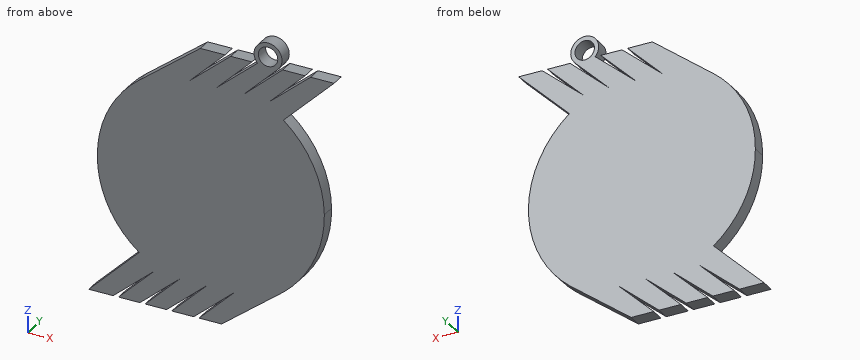
```python
from build123d import *

# Parameters (mm, degrees)
F0_R     = 2.291319
F1_DEPTH = 3.175


with BuildPart() as f1:
    # F0 (on Front) → F1 (new body)
    with BuildSketch(Plane.XZ):
        with BuildLine():
            Line((2.42887, 27.417888), (-3.408971, 27.417888))
            Line((-3.408971, 27.417888), (-17.817384, 16.07928))
            ThreePointArc((-17.817384, 16.07928), (-25.137158, 6.999169), (-27.666417, -4.386364))
            ThreePointArc((-27.666417, -4.386364), (-25.140054, -15.767724), (-17.817384, -24.839458))
            Line((-17.817384, -24.839458), (-29.714837, -36.722033))
            Line((-29.714837, -36.722033), (-23.95565, -36.722033))
            Line((-23.95565, -36.722033), (-14.339792, -28.421288))
            Line((-14.339792, -28.421288), (-22.712222, -36.722033))
            Line((-22.712222, -36.722033), (-17.655194, -36.722033))
            Line((-17.655194, -36.722033), (-8.056328, -28.420344))
            Line((-8.056328, -28.420344), (-16.424194, -36.722033))
            Line((-16.424194, -36.722033), (-11.368304, -36.722033))
            Line((-11.368304, -36.722033), (-1.727521, -28.384091))
            Line((-1.727521, -28.384091), (-10.131928, -36.722033))
            Line((-10.131928, -36.722033), (-4.964177, -36.722033))
            Line((-4.964177, -36.722033), (4.634687, -28.420345))
            Line((4.634687, -28.420345), (-3.733177, -36.722033))
            Line((-3.733177, -36.722033), (1.601154, -36.722033))
            Line((1.601154, -36.722033), (16.160648, -25.319263))
            ThreePointArc((16.160648, -25.319263), (23.359739, -15.947422), (25.809285, -4.386364))
            ThreePointArc((25.809285, -4.386364), (23.18269, 6.63908), (16.160648, 15.535728))
            Line((16.160648, 15.535728), (28.093671, 27.417888))
            Line((28.093671, 27.417888), (22.58408, 27.417888))
            Line((22.58408, 27.417888), (12.874909, 19.050129))
            Line((12.874909, 19.050129), (21.278487, 27.417888))
            Line((21.278487, 27.417888), (15.97779, 27.417888))
            Line((15.97779, 27.417888), (6.647244, 19.050129))
            Line((6.647244, 19.050129), (15.050822, 27.417888))
            Line((15.050822, 27.417888), (15.005607, 27.417888))
            ThreePointArc((15.005607, 27.417888), (12.544089, 32.902522), (10.082572, 27.417888))
            Line((10.082572, 27.417888), (10.037356, 27.417888))
            Line((10.037356, 27.417888), (0.354299, 19.050129))
            Line((0.354299, 19.050129), (8.757877, 27.417888))
            Line((8.757877, 27.417888), (3.757466, 27.417888))
            Line((3.757466, 27.417888), (-5.974708, 19.050129))
            Line((-5.974708, 19.050129), (2.42887, 27.417888))
        make_face()
        with Locations((12.544089, 29.607837)):
            Circle(F0_R, mode=Mode.SUBTRACT)
    extrude(amount=F1_DEPTH)


solid = f1.part
```
Source: CAD feature listing. Evaluate the final solid. Frame: model axes, mm. Coordinates: 2 decimals unless noted, no trailing zeros. Loops run counter-clockwise (first coordinate to the right, second up) from the corner with the lowest first, then second, coordinate; pieces in that order, holes last. Notation, with made-up numbers: M -35.5,42 L -31.5,42 A32 ccw -31.5,70 Z; hole C -24.75,46.5 d4. An arc over 180 degrees is marked long. Use a Markdown table: item, result. Add a question column.
Q1. First-contact query: pin 1 (1.6 mm diameter, centred on x = -0.5, y = -1, fed in from +Z); pin 2 (4 mm diameter, centred on x = 12.54, z = 29.61, fed in from -Y); pin 3 (6 mm diameter, centred on x = -5.5, z = 17, fed in from +Y); pin 4 (1.5 mm diameter, centred on x = 14, y = -1, fed in from -Z). Flat tips, straight axial feed; report the tip coordinate or a pass-through.
Q2. Section query A-A, the plane x = 18. Return loops of the section in (y, z) (3 decimals), and give its area (3 significant figures).
Q3. Section query D-D, the plane z = 3. Return loops of the section in (x, y) (3 decimals).
Q4. Section query B-B, the plane z = 25.5. Return loops of the section in (x, y) (3 decimals), and give its area (3 significant figures).
Q5. Material intervals for L1, parallel to Z at x = -0.5, y = -2.55; L2, parallel to X at y = -0.5, z = 23.5; L3, parallel to Z at x = -12.5, y = -2.2, sorted ascending.
Q6. Section query C-C, the plane x = -12.5. Return loops of the section in (y, z) (1 decimal).
Result:
| question | item | result |
|---|---|---|
| 1 | pin 1 | stops at z = 27.42 |
| 1 | pin 2 | passes through |
| 1 | pin 3 | stops at y = 0 |
| 1 | pin 4 | stops at z = -27.6 |
| 2 | outline | M -3.175,-23.642 L 0,-23.642 L 0,13.881 L -3.175,13.881 Z; M -3.175,17.367 L 0,17.367 L 0,23.467 L -3.175,23.467 Z; M -3.175,24.153 L 0,24.153 L 0,27.418 L -3.175,27.418 Z |
| 2 | area | 149 mm2 |
| 3 | outline | M -26.664,-3.175 L 24.622,-3.175 L 24.622,0 L -26.664,0 Z |
| 4 | outline | M -5.846,-3.175 L 0.503,-3.175 L 0.503,0 L -5.846,0 Z; M 1.527,-3.175 L 6.832,-3.175 L 6.832,0 L 1.527,0 Z; M 7.818,-3.175 L 13.125,-3.175 L 13.125,0 L 7.818,0 Z; M 13.839,-3.175 L 19.352,-3.175 L 19.352,0 L 13.839,0 Z; M 20.359,-3.175 L 26.168,-3.175 L 26.168,0 L 20.359,0 Z |
| 4 | area | 89.8 mm2 |
| 5 | L1 | z = -36.72 to -33.51, -32.86 to 23.76, 24.5 to 27.42 |
| 5 | L2 | x = -8.39 to -1.51, -0.8 to 4.82, 5.5 to 11.12, 11.61 to 17.34, 18.04 to 24.16 |
| 5 | L3 | z = -36.72 to -32.83, -32.26 to 20.26 |
| 6 | outline | M -3.2,-36.7 L 0,-36.7 L 0,-32.8 L -3.2,-32.8 Z; M -3.2,-32.3 L 0,-32.3 L 0,20.3 L -3.2,20.3 Z |
